from build123d import *

# Parameters (mm, degrees)
SKETCH1_W           = 24
SKETCH1_H           = 25
BOSS_EXTRUDE1_DEPTH = 8
SKETCH2_R           = 4
CUT_EXTRUDE1_DEPTH  = 29.217902119
SKETCH3_R           = 2.6
CUT_EXTRUDE2_DEPTH  = 20.085334684
FILLET1_R           = 3
FILLET2_R           = 5
SKETCH4_R           = 4.8
CUT_EXTRUDE3_DEPTH  = 4


with BuildPart() as part:
    # Sketch1 → Boss-Extrude1 (new body)
    with BuildSketch(Plane(origin=(0, 0, 0), x_dir=(1, 0, 0), z_dir=(0, 1, 0))):
        Rectangle(SKETCH1_W, SKETCH1_H)
    extrude(amount=BOSS_EXTRUDE1_DEPTH)

    # Sketch2 → Cut-Extrude1 (cut, through all)
    with BuildSketch(Plane.ZY.offset(12)):
        Circle(SKETCH2_R)
    extrude(amount=-CUT_EXTRUDE1_DEPTH, mode=Mode.SUBTRACT)

    # Sketch3 → Cut-Extrude2 (cut, through all)
    with BuildSketch(Plane.XZ):
        with Locations(Location((-6, -7, 0), (0, 0, 270))):
            Circle(SKETCH3_R)
        with Locations(Location((6, 7, 0), (0, 0, 270))):
            Circle(SKETCH3_R)
    extrude(amount=-CUT_EXTRUDE2_DEPTH, mode=Mode.SUBTRACT)

    # Fillet1
    # the kernel refuses this fillet: 3 mm, written as the material it takes off along each edge
    with BuildSketch(Plane(origin=(19.5, 8, 12.5), x_dir=(0, 0, -1), z_dir=(-1, 0, 0))) as fillet1_piece_1:
        with BuildLine():
            CenterArc((FILLET1_R, FILLET1_R), FILLET1_R, 180, 90)
            Line((0, FILLET1_R), (0, 0))
            Line((0, 0), (FILLET1_R, 0))
        make_face()
    extrude(amount=39, mode=Mode.SUBTRACT)
    with BuildSketch(Plane(origin=(12, 8, -20), x_dir=(0, -1, 0), z_dir=(0, 0, 1))) as fillet1_piece_2:
        with BuildLine():
            CenterArc((FILLET1_R, -FILLET1_R), FILLET1_R, 90, 90)
            Line((0, -FILLET1_R), (0, 0))
            Line((0, 0), (FILLET1_R, 0))
        make_face()
    extrude(amount=40, mode=Mode.SUBTRACT)
    with BuildSketch(Plane(origin=(-19.5, 8, -12.5), x_dir=(0, -1, 0), z_dir=(1, 0, 0))) as fillet1_piece_3:
        with BuildLine():
            CenterArc((FILLET1_R, -FILLET1_R), FILLET1_R, 90, 90)
            Line((0, -FILLET1_R), (0, 0))
            Line((0, 0), (FILLET1_R, 0))
        make_face()
    extrude(amount=39, mode=Mode.SUBTRACT)

    # Fillet2
    # the kernel refuses this fillet: 5 mm, written as the material it takes off along each edge
    with BuildSketch(Plane(origin=(7, 8, 7.5), x_dir=(0, 0, 1), z_dir=(-1, 0, 0))) as fillet2_piece_1:
        with BuildLine():
            CenterArc((2, -3), 3, 0, 90)
            Line((5, -3), (5, 0))
            Line((5, 0), (2, 0))
        make_face()
    revolve(axis=Axis((7, 8, 7.5), (0, 1, 0)), revolution_arc=90, mode=Mode.SUBTRACT)
    with BuildSketch(Plane(origin=(7, 8, -7.5), x_dir=(1, 0, 0), z_dir=(0, 0, 1))) as fillet2_piece_2:
        with BuildLine():
            CenterArc((2, -3), 3, 0, 90)
            Line((5, -3), (5, 0))
            Line((5, 0), (2, 0))
        make_face()
    revolve(axis=Axis((7, 8, -7.5), (0, 1, 0)), revolution_arc=90, mode=Mode.SUBTRACT)
    with BuildSketch(Plane(origin=(12, -12.5, -12.5), x_dir=(-1, 0, 0), z_dir=(0, 1, 0)), Plane(origin=(12, -12.5, 12.5), x_dir=(0, 0, -1), z_dir=(0, 1, 0))) as fillet2_piece_3:
        with BuildLine():
            CenterArc((FILLET2_R, FILLET2_R), FILLET2_R, 180, 90)
            Line((0, FILLET2_R), (0, 0))
            Line((0, 0), (FILLET2_R, 0))
        make_face()
    extrude(amount=20.5, mode=Mode.SUBTRACT)

    # Sketch4 → Cut-Extrude3 (cut)
    with BuildSketch(Plane(origin=(0, 8, 0), x_dir=(1, 0, 0), z_dir=(0, 1, 0))):
        with Locations(Location((-6, 7, 0), (0, 0, 270))):
            Circle(SKETCH4_R)
        with Locations(Location((6, -7, 0), (0, 0, 270))):
            Circle(SKETCH4_R)
    extrude(amount=-CUT_EXTRUDE3_DEPTH, mode=Mode.SUBTRACT)


solid = part.part
Source: CAD feature listing. Evaluate the final solid. Frame: model axes, mm. A direction names the side the tool comes from. Coordinates: 2 decimals unless noted, no trailing zeros. Loops run counter-clockwise (first coordinate to the right, second up) from the corner with the lowest first, then second, coordinate; pieces in that order, holes last. Notation, with made-up numbers: (-3, -16) - (17, -16) arc R20 cw to (17, 12) - close; hole circle Ø11 at (-37, 8). An arc over 180 degrees is marked (long way). Return JSON: item names as keys, results as strings.
Q1. Section A-A, the plane y = 1.75. Return loops of the section in (x, z).
Results:
{"outline": "(-12, -12.5) - (7, -12.5) arc R5 ccw to (12, -7.5) - (12, -3.6) - (-12, -3.6) - close; (-12, 3.6) - (12, 3.6) - (12, 7.5) arc R5 ccw to (7, 12.5) - (-12, 12.5) - close; hole circle Ø5.2 at (-6, -7); hole circle Ø5.2 at (6, 7)"}
Q2. Material intervals for line 1 along X through (y, z) = (2.75, 7); line 2 along X through (y, z) = (5.1, 7); line 3 along Z through (x, y) = (8, 6.5), sorted ascending.
Results:
{"line 1": "-12 to 3.4, 8.6 to 12", "line 2": "-12 to 1.2, 10.8 to 12", "line 3": "-11.99 to 2.64, 11.36 to 11.99"}
Q3. Section C-C, the plane x = -6. Return loops of the section in (y, z).
Results:
{"outline": "(0, -12.5) - (5, -12.5) arc R3 ccw to (6.93, -11.8) - (4, -11.8) - (4, -9.6) - (0, -9.6) - close; (0, -4.4) - (4, -4.4) - (4, -2.2) - (8, -2.2) - (8, 9.5) arc R3 ccw to (5, 12.5) - (0, 12.5) - (0, 4) arc R4 cw to (0, -4) - close"}
Q4. Section D-D, the plane y = 3. Return loops of the section in (x, z), plus the area to 3 significant figures.
Results:
{"outline": "(-12, -12.5) - (7, -12.5) arc R5 ccw to (12, -7.5) - (12, -2.65) - (-12, -2.65) - close; (-12, 2.65) - (12, 2.65) - (12, 7.5) arc R5 ccw to (7, 12.5) - (-12, 12.5) - close; hole circle Ø5.2 at (-6, -7); hole circle Ø5.2 at (6, 7)", "area": "420 mm2"}
Q5. Mould query, pull axis X, two halves, no side actions, for faces 3 (the cylindrical face through (6.78, 1.97, 4.52)), 4 (the flat face through (12, 4.7, 0.1)), 5 (the cylindrical face through (0, 4, 0)). Classes: released by +X, released by -X, zero draft, split by the parting line, or undercut.
Results:
{"face 3": "undercut", "face 4": "released by +X", "face 5": "zero draft"}
Q6. Contact query for a flat-ended pin moving along its axis: P1, Ø5, axis at x = 4, z = 6.5, coming from the +Y side. Output: stop coordinate, or through.
Results:
{"P1": "y = 4"}
Q7. Section B-B, the plane z = -7. Return loops of the section in (x, y).
Results:
{"outline": "(-12, 0) - (-8.6, 0) - (-8.6, 4) - (-10.8, 4) - (-10.8, 8) - (-12, 8) - close; (-3.4, 0) - (12, 0) - (12, 5) arc R3 ccw to (9, 8) - (-1.2, 8) - (-1.2, 4) - (-3.4, 4) - close"}
Q8. Access query for faces 1 (the cylindrical face through (10.57, 2.46, -11)), 2 (the flat face through (-8, 4, -5)). Directions: +Z, -Z, +X, -X, +Y, -Y. A direction counts if a zero-diameter tool reaches every point of the face in a straight line with its end or side. Return the directions, or none.
Results:
{"face 1": "-Z, +X, +Y, -Y", "face 2": "+Y"}
